CAD build for the part. Positions are in the model's coordinates, mm. A direction names the side the tool comes from. Coordinates: 2 decimals unless noted, no trailing zeros. Write each loop counter-clockwise with the first axis right and the second up, starting at its lowest first coordinate (ties: lowest second). Pieces come first, ordered by that corner, then holes. Notation, with made-up numbers: (-38.75, 35.25) - (18.25, 35.25) arc R19 cw to (18.25, 68.25) - close; hole circle Ø9 at (8.5, 43). An arc over 180 degrees is marked (long way). One line per question, with ' | ' between items. Start each with the question number.
1. Probe line 1 (Z direction, x = 0, y = -2.85); line 2 (X direction, y = -3.3, z = -15); line 3 (X direction, y = -1.5, z = -16.5). List the from-to ranges inside material, lowest first.
2. Band-saw the part on C-C, the plane x = -21. Write the cut outline in (y, z), then the cut area to 3 significant figures.
3. Which spindle directions (+Z, -Z, +X, -X, +Y, -Y) get a long thin tool onto all of the face, cutting with end or side? Do faces 5 (the flat face through (6, -2, -12.407)), 6 (the cylindrical face through (9.31, -1.97, 12.92)), 7 (the flat face through (-1, -4, 0)). Say none if no direction does.
4. Band-saw the part on B-B, the plane x = 0. Write the cut outline in (y, z).
5. Band-saw the part on D-D, the plane x = 13. Write the cut outline in (y, z).
6. Flat gauge pins, fed straight in: P1, Ø0.8, axis at x = 6, y = -2, coming from the +Z side; P2, Ø2, axis at x = 13.5, y = -2, coming from the +Z side; P3, Ø1.5, axis at x = -24, y = -2.5, coming from the -Z side. Where does each tip first touch, or does it go through?
7. Band-saw the part on A-A, the plane y = -1.65. Write the cut outline in (x, z), then the cut area to 3 significant figures.
8. Two-plate mould, pull along X, no slides. Class faces 1 (the cylindrical face through (34.07, -1.97, -0.62)), 2 (the cylindrical face through (9.124, -1.972, -12.898)), 3 (the cylindrical face through (30.451, -1.972, -26.655)), 4 (the flat face through (-1, 0, 0)): +X half, -X half, draft (parallel to the pull), parting line (faces both ways), or undercut.
from build123d import *

# Parameters (mm, degrees)
F0_R     = 2.5
F1_DEPTH = 4


with BuildPart() as f1:
    # F0 (on Front) → F1 (new body)
    with BuildSketch(Plane.XZ):
        with BuildLine():
            ThreePointArc((-7.989135, 12.5), (-8.11298, 12.496931), (-8.236825, 12.5))
            ThreePointArc((-8.236825, 12.5), (-9.481632, 12.904852), (-10.35122, 13.883252))
            ThreePointArc((-10.35122, 13.883252), (-31.0592, 26.345043), (-36.782912, 2.864077))
            ThreePointArc((-36.782912, 2.864077), (-34.792965, 0.702031), (-36.233629, -1.858988))
            ThreePointArc((-36.233629, -1.858988), (-31.965386, -25.974795), (-10.645566, -13.922603))
            ThreePointArc((-10.645566, -13.922603), (-9.3812, -12.524699), (-7.5, -12.407048))
            Line((-7.5, -12.407048), (-5, -12.407048))
            ThreePointArc((-5, -12.407048), (0, -17.407048), (5, -12.407048))
            Line((5, -12.407048), (7.831228, -12.407048))
            ThreePointArc((7.831228, -12.407048), (9.139477, -12.909558), (9.971767, -14.03709))
            ThreePointArc((9.971767, -14.03709), (30.817587, -26.503972), (36.182002, -2.81443))
            ThreePointArc((36.182002, -2.81443), (34.067365, -0.577316), (35.726535, 2.01566))
            ThreePointArc((35.726535, 2.01566), (31.223825, 26.147431), (10.049361, 13.727334))
            ThreePointArc((10.049361, 13.727334), (9.295627, 12.909806), (8.261931, 12.5))
            ThreePointArc((8.261931, 12.5), (7.880498, 12.47073), (7.499065, 12.5))
            Line((7.499065, 12.5), (4.85588, 12.5))
            ThreePointArc((4.85588, 12.5), (-0.14412, 17.5), (-5.14412, 12.5))
            Line((-5.14412, 12.5), (-7.989135, 12.5))
        make_face()
        with Locations((0, -12.407048)):
            Circle(F0_R, mode=Mode.SUBTRACT)
        with Locations((-0.14412, 12.5)):
            Circle(F0_R, mode=Mode.SUBTRACT)
    extrude(amount=F1_DEPTH)


solid = f1.part
Filled in:
1) line 1: z = -17.41 to -14.91, -9.91 to 10, 15 to 17.5 | line 2: x = -40.34 to -10.79, -4.28 to 4.28, 10.09 to 39.74 | line 3: x = -40 to -11.14, -2.87 to 2.87, 10.4 to 39.43
2) outline: (-4, -26.69) - (0, -26.69) - (0, 26.87) - (-4, 26.87) - close | area: 214 mm²
3) face 5: -Z, +Y, -Y | face 6: +Z, +Y, -Y | face 7: +Z, -Z, +X, -X, -Y
4) outline: (-4, -17.41) - (0, -17.41) - (0, -14.91) - (-4, -14.91) - close; (-4, -9.91) - (0, -9.91) - (0, 10) - (-4, 10) - close; (-4, 15) - (0, 15) - (0, 17.5) - (-4, 17.5) - close
5) outline: (-4, -21.83) - (0, -21.83) - (0, 21.5) - (-4, 21.5) - close
6) P1: stops at z = 12.5 | P2: stops at z = 23.21 | P3: stops at z = -27.38
7) outline: (-36.78, 2.86) arc R2.5 cw to (-36.23, -1.86) arc R15 ccw (long way) to (-10.65, -13.92) arc R2.5 cw to (-7.5, -12.41) - (-5, -12.41) arc R5 ccw to (5, -12.41) - (7.83, -12.41) arc R2.5 cw to (9.97, -14.04) arc R15 ccw (long way) to (36.18, -2.81) arc R2.5 cw to (35.73, 2.02) arc R15 ccw (long way) to (10.05, 13.73) arc R2.5 cw to (8.26, 12.5) arc R2.5 cw to (7.5, 12.5) - (4.86, 12.5) arc R5 ccw to (-5.14, 12.5) - (-7.99, 12.5) arc R2.5 cw to (-8.24, 12.5) arc R2.5 cw to (-10.35, 13.88) arc R15 ccw (long way) to start; hole circle Ø5 at (-0.14, 12.5); hole circle Ø5 at (0, -12.41) | area: 3,370 mm²
8) face 1: +X half | face 2: undercut | face 3: undercut | face 4: draft
